Autodesk Inventor part; units mm, degrees
ref_plane "YZ Plane" through (0, 0, 0) normal (1, 0, 0) x (0, 1, 0)
ref_plane "XZ Plane" through (0, 0, 0) normal (0, 1, 0) x (-1, 0, 0)
ref_plane "XY Plane" through (0, 0, 0) normal (0, 0, 1) x (1, 0, 0)
sketch "Sketch1" plane through (0, 0, 0) normal (0, 0, 1) x (1, 0, 0)
  line L0 (0, 0) -> (72.4, 0)
  line L1 (72.4, 0) -> (72.4, 71)
  line L2 (72.4, 71) -> (0, 71)
  line L3 (0, 71) -> (0, 0)
  dimension "d0" = 72.4
  dimension "d1" = 71
extrude "Extrusion1" add sketch "Sketch1" along normal blind 10
sketch "Sketch2" plane through (0, 0, 10) normal (0, 0, 1) x (1, 0, 0)
  line L0 (72.4, 0) -> (72.4, 71)
  line L1 (72.4, 15.5) -> (82.4, 15.5)
  line L2 (82.4, 15.5) -> (82.4, 55.5)
  line L3 (82.4, 55.5) -> (72.4, 55.5)
  line L4 (72.4, 55.5) -> (72.4, 15.5)
  line L5 (72.4, 71) -> (0, 71)
  circle A0 centre (77.4, 35.5) radius 2.5
  line L6 (0, 0) -> (72.4, 0)
  point P0 (82.4, 35.5)
  point P1 (77.4, 55.5)
  dimension "d4" = 10
  dimension "d5" = 40
  dimension "d7" = 5
  dimension "d31" = 15.5
extrude "Extrusion2" add sketch "Sketch2" against normal blind 10
sketch "Sketch3" plane through (0, 0, 10) normal (0, 0, 1) x (1, 0, 0)
  line L0 (72.4, 55.5) -> (82.4, 55.5)
  line L1 (72.4, 15.5) -> (82.4, 15.5)
  line L2 (82.4, 55.5) -> (72.4, 55.5)
  line L3 (72.4, 55.5) -> (72.4, 15.5)
  line L4 (72.4, 15.5) -> (82.4, 15.5)
  line L5 (82.4, 15.5) -> (82.4, 55.5)
  point P0 (0, 0)
extrude "Extrusion3" cut sketch "Sketch3" against normal blind 5
sketch "Sketch8" plane through (0, 0, 0) normal (0, 0, -1) x (-1, 0, 0)
  line L0 (-12.4, 10) -> (-52.4, 10)
  line L1 (-52.4, 10) -> (-52.4, 0)
  line L2 (-52.4, 0) -> (-12.4, 0)
  line L3 (-12.4, 0) -> (-12.4, 10)
  line L4 (0, 0) -> (-72.4, 0)
  line L5 (-72.4, 0) -> (-72.4, 15.5)
  line L6 (-72.4, 71) -> (0, 71)
  point P0 (-36.2, 0)
  point P1 (-32.4, 10)
  point P2 (-32.4, 0)
  dimension "d32" = 40
  dimension "d33" = 10
  dimension "d34" = 20
extrude "Extrusion8" cut sketch "Sketch8" against normal blind 5
sketch "Sketch9" plane through (0, 0, 5) normal (0, 0, -1) x (-1, 0, 0)
  line L0 (-52.4, 0) -> (-52.4, 10) construction
  line L1 (-12.4, 10) -> (-12.4, 0) construction
  circle A0 centre (-32.4, 5) radius 2.5
  line L2 (-52.4, 10) -> (-12.4, 10)
  line L3 (-12.4, 0) -> (-52.4, 0)
  point P0 (0, 0)
  point P1 (-32.4, 0)
  point P2 (-12.4, 5)
  dimension "d37" = 5
extrude "Extrusion9" cut sketch "Sketch9" against normal through all
sketch "Sketch10" plane through (0, 0, 0) normal (0, 0, -1) x (-1, 0, 0)
  line L0 (0, 71) -> (0, 0)
  line L1 (0, 15.5) -> (10, 15.5)
  line L2 (10, 15.5) -> (10, 55.5)
  line L3 (10, 55.5) -> (0, 55.5)
  line L4 (0, 55.5) -> (0, 15.5)
  circle A0 centre (5, 35.5) radius 2.5
  point P0 (-82.4, 15.5)
  point P1 (10, 35.5)
  point P2 (5, 15.5)
  dimension "d40" = 10
  dimension "d41" = 40
  dimension "d42" = 5
extrude "Extrusion10" add sketch "Sketch10" against normal blind 5
properties part number "SP002" material "ABS Plastic"
Read the model definition and answer for the solid it produces. Units are mm, in the model's axes. A direction names the side the tool comes from. Give positions to 0.01 mm unless a question says otherwise; leave off trailing zeros. Order: outer loops, then holes, each group sorted by start corner. A loop starts at its lowest first (then second) coordinate and runs counter-clockwise, first axis right, second up. Notation, with made-up numbers: (10.5, 37.5) -> (46.5, 37.5) arc R25 cw to (46.5, 49.5) -> close; hole circle Ø6 at (39.25, 39). An arc over 180 degrees is marked (long way). One line per item, written item: value. Start each with the question number.
(1) For a pull along Y with two mould halves and no side action, classify faces 1 (the flat face through (36, 36, 10)), 2 (the flat face through (-5, 15.5, 2)), 3 (the cylindrical face through (34.9, 5.1, 7.5)) as released by +Y, released by -Y, zero draft, split by the parting line, or undercut.
(2) A tool of negligible diameter and unlimited length cuts with its end or side. For faces 4 (the flat face through (-8, 36, 5)), 5 (the flat face through (33, 8, 5)), 6 (the flat face through (74, 36, 5)), 7 (the flat face through (-5, 55.5, 2)), 8 (the flat face through (77, 55.5, 3)), from which of +Z, -Z, +X, -X, +Y, -Y can it reach the whole face along a straight path? Write none if from no direction.
(3) Straight lines are drawn through the part: L1, parallel to X at y = 6, z = 0.5; L2, parallel to Y at x = 77.4, z = 1.3; L3, parallel to Y at x = 23, z = 4.75. For each, find the intervals that lie inside material, in ascending order.
(4) Flat-ended cylindrical pins translate along their axes: P1, Ø5.5, axis at y = 7, z = 2, coming from the -X side; P2, Ø6, axis at x = 32.4, y = 5, coming from the +Z side; P3, Ø2.5, axis at x = -7, z = 3.5, coming from the -Y side; P4, Ø4, axis at y = 6.5, z = 3.5, coming from the +X side. Find the tip coordinate at first contact, or state that the pin passes through.
(5) The part is cut by section B-B (y = 5). Determine the outline of the cut face in (x, z).
(6) The part is cut by section C-C (y = 35.5). Determine the outline of the cut face in (x, z).
(7) The part is cut by section D-D (z = 7). Determine the outline of the cut face in (x, y).
(8) The part is cut by section A-A (x = 77.4). Determine the outline of the cut face in (y, z), and give its area (3 significant figures).
Taken from the geometry:
1. face 1: zero draft
1. face 2: released by -Y
1. face 3: undercut
2. face 4: +Z, -X, +Y, -Y
2. face 5: -Z, -Y
2. face 6: +Z, +X, +Y, -Y
2. face 7: +Z, -Z, -X, +Y
2. face 8: +Z, -Z, +X, +Y
3. L1: 0 to 12.4, 52.4 to 72.4
3. L2: 15.5 to 33, 38 to 55.5
3. L3: 10 to 71
4. P1: x = 0
4. P2: z = 10
4. P3: y = 15.5
4. P4: x = 72.4
5. outline: (0, 0) -> (12.4, 0) -> (12.4, 5) -> (29.9, 5) -> (29.9, 10) -> (0, 10) -> close; (34.9, 5) -> (52.4, 5) -> (52.4, 0) -> (72.4, 0) -> (72.4, 10) -> (34.9, 10) -> close
6. outline: (-10, 0) -> (-7.5, 0) -> (-7.5, 5) -> (-10, 5) -> close; (-2.5, 0) -> (74.9, 0) -> (74.9, 5) -> (72.4, 5) -> (72.4, 10) -> (0, 10) -> (0, 5) -> (-2.5, 5) -> close; (79.9, 0) -> (82.4, 0) -> (82.4, 5) -> (79.9, 5) -> close
7. outline: (0, 0) -> (72.4, 0) -> (72.4, 71) -> (0, 71) -> close; hole circle Ø5 at (32.4, 5)
8. outline: (15.5, 0) -> (33, 0) -> (33, 5) -> (15.5, 5) -> close; (38, 0) -> (55.5, 0) -> (55.5, 5) -> (38, 5) -> close
8. area: 175 mm^2
